Model file for the job. Use its own axes, mm. Give positions to 0.01 mm unless a question says otherwise; leave off trailing zeros. Write each loop counter-clockwise with the first axis right and the second up, starting at its lowest first coordinate (ties: lowest second). Pieces come first, ordered by that corner, then holes. Notation, with made-up numbers: (-13, -11.75) - (46, -11.75) arc R12 ccw to (46, 3.25) - close; hole circle Ø7 at (28, 22). An arc over 180 degrees is marked (long way). One line per item, written item: value. Start each with the question number.
(1) Cut at D-D, the plane y = 15. List the corners of the cut face in (x, z).
(2) Probe L1, parallel to Y at x = 0, z = 2.95; L2, parallel to Y at x = -19, z = 4.7; L3, parallel to Y at x = 16, z = 1.4. List the from-to ranges inside material, lowest first.
(3) Cut at A-A, the plane x = 0. List the corners of the cut face in (y, z), and give its area (3 significant figures).
(4) Drop a flat-ended pin along its axis: P1, Ø1, axis at y = -37.5, z = 3, coming from the -X side. Give the stop position or say it passes through.
(5) Cut at C-C, the plane y = -30. List the corners of the cut face in (x, z).
(6) Cut at B-B, the plane y = 0. List the corners of the cut face in (x, z).
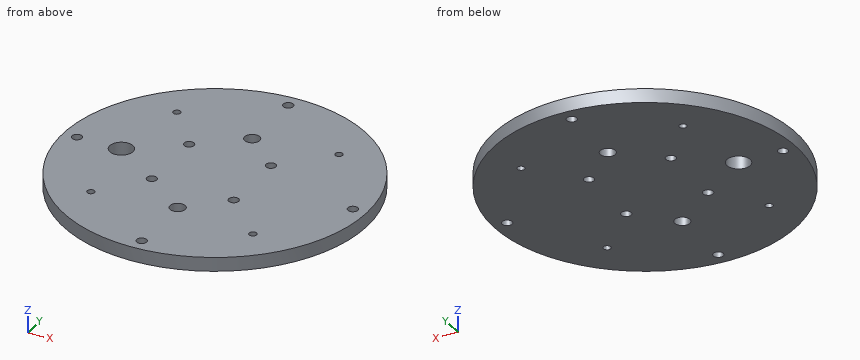
from build123d import *

# Parameters (mm, degrees)
SKETCH_1_R      = 65
SKETCH_1_R_2    = 1.6
SKETCH_1_R_3    = 2.15
SKETCH_1_R_4    = 3.25
SKETCH_1_R_5    = 5
EXTRUDE_1_DEPTH = 6


with BuildPart() as part:
    # 草圖1 → 填料-伸長1 (new body)
    with BuildSketch(Plane.XY):
        Circle(SKETCH_1_R)
        with Locations((34.648232278, 34.648232278)):
            Circle(SKETCH_1_R_2, mode=Mode.SUBTRACT)
        with Locations((-34.648232278, 34.648232278)):
            Circle(SKETCH_1_R_2, mode=Mode.SUBTRACT)
        with Locations((-34.648232278, -34.648232278)):
            Circle(SKETCH_1_R_2, mode=Mode.SUBTRACT)
        with Locations((34.648232278, -34.648232278)):
            Circle(SKETCH_1_R_2, mode=Mode.SUBTRACT)
        with Locations((59, 0)):
            Circle(SKETCH_1_R_3, mode=Mode.SUBTRACT)
        with Locations((0, 59)):
            Circle(SKETCH_1_R_3, mode=Mode.SUBTRACT)
        with Locations((-59, 0)):
            Circle(SKETCH_1_R_3, mode=Mode.SUBTRACT)
        with Locations((0, -59)):
            Circle(SKETCH_1_R_3, mode=Mode.SUBTRACT)
        with Locations((-19, 15)):
            Circle(SKETCH_1_R_3, mode=Mode.SUBTRACT)
        with Locations((-19, -15)):
            Circle(SKETCH_1_R_3, mode=Mode.SUBTRACT)
        with Locations((16, 15)):
            Circle(SKETCH_1_R_3, mode=Mode.SUBTRACT)
        with Locations((16, -15)):
            Circle(SKETCH_1_R_3, mode=Mode.SUBTRACT)
        with Locations((0, 30)):
            Circle(SKETCH_1_R_4, mode=Mode.SUBTRACT)
        with Locations((0, -30)):
            Circle(SKETCH_1_R_4, mode=Mode.SUBTRACT)
        with Locations((-40, 0)):
            Circle(SKETCH_1_R_5, mode=Mode.SUBTRACT)
    extrude(amount=EXTRUDE_1_DEPTH)


solid = part.part
Answers follow:
1. outline: (-63.25, 0) - (-21.15, 0) - (-21.15, 6) - (-63.25, 6) - close; (-16.85, 0) - (13.85, 0) - (13.85, 6) - (-16.85, 6) - close; (18.15, 0) - (63.25, 0) - (63.25, 6) - (18.15, 6) - close
2. L1: y = -65 to -61.15, -56.85 to -33.25, -26.75 to 26.75, 33.25 to 56.85, 61.15 to 65
2. L2: y = -62.16 to -17.15, -12.85 to 12.85, 17.15 to 62.16
2. L3: y = -63 to -17.15, -12.85 to 12.85, 17.15 to 63
3. outline: (-65, 0) - (-61.15, 0) - (-61.15, 6) - (-65, 6) - close; (-56.85, 0) - (-33.25, 0) - (-33.25, 6) - (-56.85, 6) - close; (-26.75, 0) - (26.75, 0) - (26.75, 6) - (-26.75, 6) - close; (33.25, 0) - (56.85, 0) - (56.85, 6) - (33.25, 6) - close; (61.15, 0) - (65, 0) - (65, 6) - (61.15, 6) - close
3. area: 650 mm²
4. P1: stops at x = -53.44
5. outline: (-57.66, 0) - (-3.25, 0) - (-3.25, 6) - (-57.66, 6) - close; (3.25, 0) - (57.66, 0) - (57.66, 6) - (3.25, 6) - close
6. outline: (-65, 0) - (-61.15, 0) - (-61.15, 6) - (-65, 6) - close; (-56.85, 0) - (-45, 0) - (-45, 6) - (-56.85, 6) - close; (-35, 0) - (56.85, 0) - (56.85, 6) - (-35, 6) - close; (61.15, 0) - (65, 0) - (65, 6) - (61.15, 6) - close
